Here's the drawing with two shaded views (mm, measured from the low corner). I have some questions. A direction names the side the tool comes from. Coordinates: 2 decimals unless noted, no trailing zeros. Order: outer loops, then holes, each group sorted by start corner. A loop starts at its lowest first (then second) coordinate and runs counter-clockwise, first axis right, second up. Notation, with made-up numbers: (65.25, -9) -> (89.25, -9) arc R14 cw to (89.25, 0) -> close; hole circle Ø3 at (22, -29.75). An arc over 180 degrees is marked (long way). Answer in a Markdown table with one row per item. Add a question column.
1. Imagine slicing it at B-B on y = 8. Write out the boundary of the cut face in (x, z).
2. If I drill on line 1 along Z through (x, y) = (11.75, 12.75); line 2 along Y through (x, z) = (8.75, 0.75) (1 decimal); line 3 along X through (y, z) = (8, 3.75), over which ranges is the centre line in solid material (lowest first)? Write a range as [from, to].
3. Imagine slicing it at D-D on x = 13.5. Write out the boundary of the cut face in (y, z).
4. Will these pins go through, and if not, where does the flat tip stop? pin 1 (8 mm diameter, centred on x = 5.5, y = 6.5, fed in from -Z); pin 2 (0.6 mm diameter, centred on x = 8.5, y = 14.5, fed in from -Z); pin 3 (1.5 mm diameter, centred on x = 12, z = 8.5, fed in from +Y); pin 4 (5 mm diameter, centred on x = 8, y = 8, fed in from +Z).
5. Imagine slicing it at C-C on z = 3. Write out the boundary of the cut face in (x, y).
6. On a 3-axis mill with a long thin cutter (end or side, diameter ignored), from which of +Z, -Z, +X, -X, +Y, -Y can I reach the whole of each face in a straight line? I mean the marked faces 4 and 5. Say none if no direction works.
7. We'd pull the mould along X, two halves only. Please class the marked faces 1, 2 and 3: pulls with the +X half, pulls with the -X half, needs draft (parallel to the pull), parting line crosses it, or undercut.
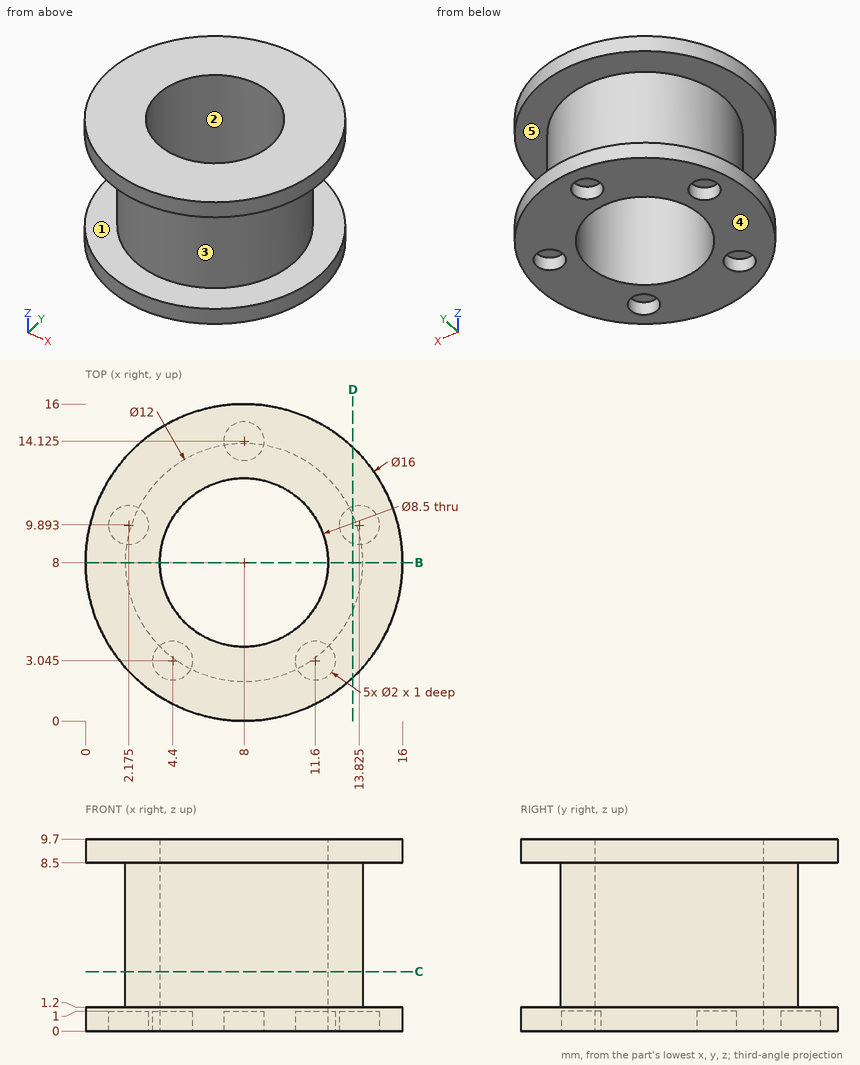
Answers follow:
| question | item | result |
|---|---|---|
| 1 | outline | (0, 0) -> (3.75, 0) -> (3.75, 9.7) -> (0, 9.7) -> (0, 8.5) -> (2, 8.5) -> (2, 1.2) -> (0, 1.2) -> close; (12.25, 0) -> (16, 0) -> (16, 1.2) -> (14, 1.2) -> (14, 8.5) -> (16, 8.5) -> (16, 9.7) -> (12.25, 9.7) -> close |
| 2 | line 1 | z = [0, 1.2], [8.5, 9.7] |
| 2 | line 2 | y = [0, 3.8], [12.2, 13.5], [14.8, 16] |
| 2 | line 3 | x = [2, 3.75], [12.25, 14] |
| 3 | outline | (2.19, 0) -> (8.95, 0) -> (8.95, 1) -> (10.84, 1) -> (10.84, 0) -> (13.81, 0) -> (13.81, 1.2) -> (10.4, 1.2) -> (10.4, 8.5) -> (13.81, 8.5) -> (13.81, 9.7) -> (2.19, 9.7) -> (2.19, 8.5) -> (5.6, 8.5) -> (5.6, 1.2) -> (2.19, 1.2) -> close |
| 4 | pin 1 | stops at z = 0 |
| 4 | pin 2 | stops at z = 1 |
| 4 | pin 3 | stops at y = 15.31 |
| 4 | pin 4 | passes through |
| 5 | outline | circle Ø12 at (8, 8); hole circle Ø8.5 at (8, 8) |
| 6 | face 4 | -Z, +X, -X, +Y, -Y |
| 6 | face 5 | none |
| 7 | face 1 | needs draft |
| 7 | face 2 | undercut |
| 7 | face 3 | parting line crosses it |
